The listing builds one solid part. Answer for the finished solid, in the listing's coordinates (mm). A direction names the side the tool comes from. Coordinates: 2 decimals unless noted, no trailing zeros. Write each loop counter-clockwise with the first axis right and the second up, starting at its lowest first coordinate (ties: lowest second). Pieces come first, ordered by that corner, then holes. Notation, with made-up numbers: M -32.5,80.25 L 2.5,80.25 A8 cw 2.5,85.25 Z; hole C 46.25,45 d10. An arc over 180 degrees is marked long. Write item = value, one per line. Start each with the question number.
```python
from build123d import *

# Parameters (mm, degrees)
F0_R     = 9.525
F1_DEPTH = 7.62


with BuildPart() as f1:
    # F0 (on Top) → F1 (new body)
    with BuildSketch(Plane.XY):
        with BuildLine():
            ThreePointArc((71.507275, -26.327734), (62.992, 0), (71.507275, 26.327734))
            ThreePointArc((71.507275, 26.327734), (69.990436, 30.129369), (68.271654, 33.844073))
            Line((68.271654, 33.844073), (40.687859, 17.918561))
            ThreePointArc((40.687859, 17.918561), (34.09542, 19.685), (35.861859, 26.277439))
            Line((35.861859, 26.277439), (63.445654, 42.20295))
            ThreePointArc((63.445654, 42.20295), (61.088017, 45.548811), (58.554124, 48.76325))
            ThreePointArc((58.554124, 48.76325), (31.496, 54.552672), (12.953151, 75.090984))
            ThreePointArc((12.953151, 75.090984), (8.902419, 75.67818), (4.826, 76.047023))
            Line((4.826, 76.047023), (4.826, 44.196))
            ThreePointArc((4.826, 44.196), (0, 39.37), (-4.826, 44.196))
            Line((-4.826, 44.196), (-4.826, 76.047023))
            ThreePointArc((-4.826, 76.047023), (-8.902419, 75.67818), (-12.953151, 75.090984))
            ThreePointArc((-12.953151, 75.090984), (-31.496, 54.552672), (-58.554124, 48.76325))
            ThreePointArc((-58.554124, 48.76325), (-61.088017, 45.548811), (-63.445654, 42.20295))
            Line((-63.445654, 42.20295), (-35.861859, 26.277439))
            ThreePointArc((-35.861859, 26.277439), (-34.09542, 19.685), (-40.687859, 17.918561))
            Line((-40.687859, 17.918561), (-68.271654, 33.844073))
            ThreePointArc((-68.271654, 33.844073), (-69.990436, 30.129369), (-71.507275, 26.327734))
            ThreePointArc((-71.507275, 26.327734), (-62.992, 0), (-71.507275, -26.327734))
            ThreePointArc((-71.507275, -26.327734), (-69.990436, -30.129369), (-68.271654, -33.844073))
            Line((-68.271654, -33.844073), (-40.687859, -17.918561))
            ThreePointArc((-40.687859, -17.918561), (-34.09542, -19.685), (-35.861859, -26.277439))
            Line((-35.861859, -26.277439), (-63.445654, -42.20295))
            ThreePointArc((-63.445654, -42.20295), (-61.088017, -45.548811), (-58.554124, -48.76325))
            ThreePointArc((-58.554124, -48.76325), (-31.496, -54.552672), (-12.953151, -75.090984))
            ThreePointArc((-12.953151, -75.090984), (-8.902419, -75.67818), (-4.826, -76.047023))
            Line((-4.826, -76.047023), (-4.826, -44.196))
            ThreePointArc((-4.826, -44.196), (0, -39.37), (4.826, -44.196))
            Line((4.826, -44.196), (4.826, -76.047023))
            ThreePointArc((4.826, -76.047023), (8.902419, -75.67818), (12.953151, -75.090984))
            ThreePointArc((12.953151, -75.090984), (31.496, -54.552672), (58.554124, -48.76325))
            ThreePointArc((58.554124, -48.76325), (61.088017, -45.548811), (63.445654, -42.20295))
            Line((63.445654, -42.20295), (35.861859, -26.277439))
            ThreePointArc((35.861859, -26.277439), (34.09542, -19.685), (40.687859, -17.918561))
            Line((40.687859, -17.918561), (68.271654, -33.844073))
            ThreePointArc((68.271654, -33.844073), (69.990436, -30.129369), (71.507275, -26.327734))
        make_face()
        Circle(F0_R, mode=Mode.SUBTRACT)
    extrude(amount=F1_DEPTH)


solid = f1.part
```
1. Each of these flat-tipped pins is pushed along its axis until it touches: pin 1 (4 mm diameter, centred on y = 31, z = 5.5, fed in from -X); pin 2 (3 mm diameter, centred on y = -48.5, z = 4, fed in from +X); pin 3 (4 mm diameter, centred on y = 64.5, z = 2.5, fed in from +X). Where does it stop, or does it pass through?
2. The part is cut by section D-D, the plane x = -22.5. Write down the section's boundary in (y, z), and give its area (3 significant figures).
3. Straight lines are drawn through the part: L1, parallel to Y at x = 0, z = 2.5 (3 decimals); L2, parallel to Y at x = 57, z = 4.25; L3, parallel to Y at x = 51, z = 5.25. For each, find the intervals that lie inside material, in ascending order. Write a range as [from, to].
4. The part is cut by section A-A, the plane x = 0. Write down the section's boundary in (y, z) (3 decimals).
5. For a pull along Y with two mould halves and no side action, classify faces 1 (the face through (-8.96, -75.67, 3.76)), 2 (the face through (4.826, 60, 4)), 3 (the face through (-54.67, -25.99, 3.76)), 4 (the face through (49.46, 34.13, 3.76)) as pulls with the +Y half, pulls with the -Y half, needs draft (parallel to the pull), parting line crosses it, or undercut.
6. The part is cut by section C-C, the plane x = -48. Write down the section's boundary in (y, z).
7. For faces 5 (the face through (4.826, -60, 4)), 6 (the face through (54.29, -25.77, 3.76)), 7 (the face through (61.054, -45.595, 3.757)), determine the directions among +Z, -Z, +X, -X, +Y, -Y from which every point of the face is accessible in a straight line to the end or side of a thin tool.
8. The part is cut by section B-B, the plane y = 0. Write down the section's boundary in (x, z) (3 decimals).
Solution:
q1.pin_1 = -70.47
q1.pin_2 = 59.98
q1.pin_3 = 21.4
q2.outline = M -61.39,0 L 61.39,0 L 61.39,7.62 L -61.39,7.62 Z
q2.area = 936 mm^2
q3.L1 = [-39.37, -9.525], [9.525, 39.37]
q3.L2 = [-48.63, -38.48], [-27.34, 27.34], [38.48, 48.63]
q3.L3 = [-48.63, -35.02], [-23.87, 23.87], [35.02, 48.63]
q4.outline = M -39.37,0 L -9.525,0 L -9.525,7.62 L -39.37,7.62 Z; M 9.525,0 L 39.37,0 L 39.37,7.62 L 9.525,7.62 Z
q5.face_1 = pulls with the -Y half
q5.face_2 = needs draft
q5.face_3 = undercut
q5.face_4 = undercut
q6.outline = M -48.93,0 L -33.29,0 L -33.29,7.62 L -48.93,7.62 Z; M -22.14,0 L 22.14,0 L 22.14,7.62 L -22.14,7.62 Z; M 33.29,0 L 48.93,0 L 48.93,7.62 L 33.29,7.62 Z
q7.face_5 = +Z, -Z, -Y
q7.face_6 = +Z, -Z
q7.face_7 = +Z, -Z, +X, -Y
q8.outline = M -62.992,0 L -9.525,0 L -9.525,7.62 L -62.992,7.62 Z; M 9.525,0 L 62.992,0 L 62.992,7.62 L 9.525,7.62 Z
